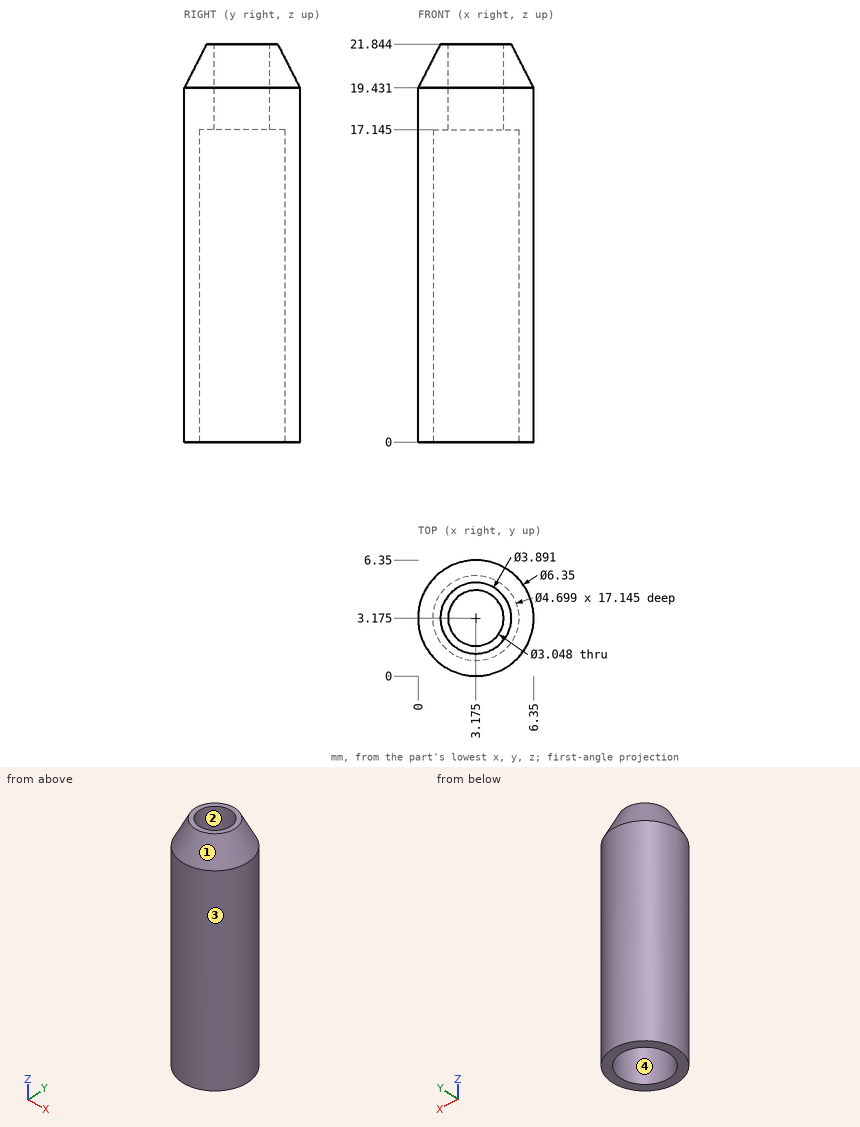
Answer from the drawing. Dimensions are ordinates in mm from the lowest x, y and z of the part. A direction names the side the tool comes from. Coordinates: 2 decimals unless noted, no trailing zeros. One line per question, with ' | ' between items.
Q1. For the marked faces 3 and 4, determine the directions among +Z, -Z, +X, -X, +Y, -Y from which every point of the face is accessible in a straight line to the end or side of a thin tool.
Result set:
face 3: +Z, -Z | face 4: -Z
Q2. Determine the mould class of the marked faces 1 and 2 for opening direction Y: +Y half, -Y half, draft (parallel to the pull), parting line (faces both ways), or undercut.
Result set:
face 1: parting line | face 2: undercut
Q3. Each of these flat-tipped pins is pushed along its axis until it touches: P1, Ø3, axis at x = 5, z = 17, coming from the +Y side; P2, Ø1, axis at y = 5, z = 7, coming from the -X side; P3, Ø1, axis at y = 5, z = 11.5, coming from the +X side. Where does it stop, or does it pass through?
Result set:
P1: y = 6.33 | P2: x = 0.29 | P3: x = 6.06
Q4. Consider L1, parallel to X at y = 3.5, z = 15.5; L2, parallel to Y at x = 5.25, z = 6.5. Determine where each line is inside the solid, lowest interval first. Write a range as [from, to].
Result set:
L1: [0.02, 0.85], [5.5, 6.33] | L2: [0.77, 2.07], [4.28, 5.58]
